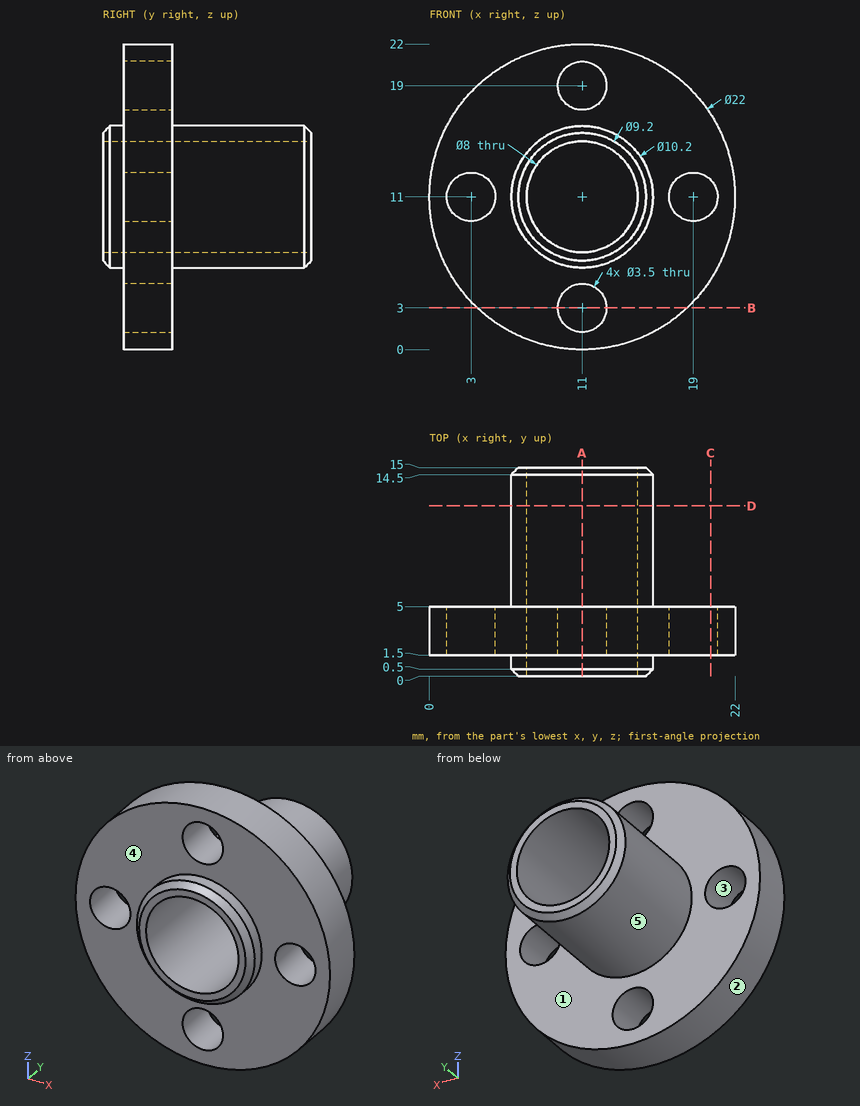
Design review of the part shown in the three views and the two pictorial views. Dimensions are in mm from the part's minimum x, y and z. A direction names the side the tool comes from. Round coordinates to 2 decimals unless told otherwise and drop trailing zeros. Order: outer loops, then holes, each group sorted by start corner. A loop starts at its lowest first (then second) coordinate and runs counter-clockwise, first axis right, second up.
Item 1: Machinability: for the marked faces 1 and 2, which of the approach directions +Z, -Z, +X, -X, +Y, -Y give a long, thin tool a straight path to every point of the face, cutting with its end or side? Answer none if there is none.
Working result:
face 1: +Y
face 2: +Y, -Y
Item 2: Add section D-D, the plane y = 12.25. State the section outline as (x, z) points, and give its area (3 significant figures).
Working result:
outline: circle Ø10.2 at (11, 11); hole circle Ø8 at (11, 11)
area: 31.4 mm2
Item 3: For pin 1 (3 mm diameter, centred on x = 18.5, z = 3.5, fed in from -Y); pin 2 (1.5 mm diameter, centred on x = 3.5, y = 8, fed in from +Z); pin 3 (6 mm diameter, centred on y = 8.5, z = 12, fed in from +X); pin 4 (1.5 mm diameter, centred on x = 14, y = 4, fed in from +Z), all flat-tipped, find the tip position at first contact; note any pin that passes through.
Working result:
pin 1: stops at y = 1.5
pin 2: passes through
pin 3: stops at x = 16.1
pin 4: stops at z = 21.77
Item 4: Add section A-A, the plane x = 11. State the section outline as (y, z) points.
Working result:
outline: (0, 6.4) - (0.5, 5.9) - (1.5, 5.9) - (1.5, 4.75) - (5, 4.75) - (5, 5.9) - (14.5, 5.9) - (15, 6.4) - (15, 7) - (0, 7) - close; (0, 15) - (15, 15) - (15, 15.6) - (14.5, 16.1) - (5, 16.1) - (5, 17.25) - (1.5, 17.25) - (1.5, 16.1) - (0.5, 16.1) - (0, 15.6) - close; (1.5, 0) - (5, 0) - (5, 1.25) - (1.5, 1.25) - close; (1.5, 20.75) - (5, 20.75) - (5, 22) - (1.5, 22) - close
Item 5: Add section B-B, the plane z = 3. State the section outline as (x, y) points.
Working result:
outline: (3.45, 1.5) - (9.25, 1.5) - (9.25, 5) - (3.45, 5) - close; (12.75, 1.5) - (18.55, 1.5) - (18.55, 5) - (12.75, 5) - close
Item 6: To check wall thickness, follow probe 1 along X at (y, z) = (6, 11); probe 2 along Y at (x, z) = (8.75, 4); probe 3 along X at (y, z) = (4.25, 4.5). State the ranges of each line that lie inside material, in increasing order.
Working result:
probe 1: x = 5.9 to 7, 15 to 16.1
probe 2: y = 1.5 to 5
probe 3: x = 2.13 to 10.1, 11.9 to 19.87
Item 7: Add section C-C, the plane x = 20.25. State the section outline as (y, z) points.
Working result:
outline: (1.5, 5.05) - (5, 5.05) - (5, 9.78) - (1.5, 9.78) - close; (1.5, 12.22) - (5, 12.22) - (5, 16.95) - (1.5, 16.95) - close
Item 8: Draft analysis for pull direction X (two halves, no side actions). For the marked faces 3, 4 and 5, state which applies: released by +X, released by -X, zero draft, split by the parting line, or undercut.
Working result:
face 3: undercut
face 4: zero draft
face 5: split by the parting line
